Verification items for the finished model (mm, model axes). A direction names the side the tool comes from. Coordinates: 2 decimals unless noted, no trailing zeros. Order: outer loops, then holes, each group sorted by start corner. A loop starts at its lowest first (then second) coordinate and runs counter-clockwise, first axis right, second up. Notation, with made-up numbers: M 45.25,-10.5 L 84.25,-10.5 A33 ccw 84.25,20.5 Z; hole C -39,-40 d10. An arc over 180 degrees is marked long. Use one line per item in the form item = value. Start each with the question number.
```python
from build123d import *

# Parameters (mm, degrees)
F1_DEPTH = 6.35
F0_W     = 3.81
F0_H     = 76.2000009209
F0_H_2   = 76.2
F2_DEPTH = 3.175


# Not quite as in the source:
# - ends of sketch curves that miss each other by under 0.0002 mm in the source are joined


with BuildPart() as f1:
    # F0 (on Top) → F1 (new body, symmetric)
    with BuildSketch(Plane.XY):
        with BuildLine():
            Line((-49.2071506187, 28.1480993807), (-49.2071506187, 21.7980993807))
            Line((-49.2071506187, 21.7980993807), (-45.3971506187, 21.7980993807))
            Line((-45.3971506187, 21.7980993807), (-26.2557423981, 21.7980993807))
            Line((-26.2557423981, 21.7980993807), (-22.4457423981, 21.7980993807))
            Line((-22.4457423981, 21.7980993807), (-1.3203332201, 21.7980993807))
            Line((-1.3203332201, 21.7980993807), (2.4896667799, 21.7980993807))
            Line((2.4896667799, 21.7980993807), (21.6630548239, 21.7980993807))
            Line((21.6630548239, 21.7980993807), (25.4730548239, 21.7980993807))
            Line((25.4730548239, 21.7980993807), (45.6722128358, 21.7980993807))
            Line((45.6722128358, 21.7980993807), (49.4822128358, 21.7980993807))
            Line((49.4822128358, 21.7980993807), (49.8528493813, 21.7980993807))
            Line((49.8528493813, 21.7980993807), (49.8528493813, 28.1480993807))
            ThreePointArc((49.8528493813, 28.1480993807), (47.9929774418, 32.6382274413), (43.5028493813, 34.4980993807))
            Line((43.5028493813, 34.4980993807), (-42.8571506187, 34.4980993807))
            ThreePointArc((-42.8571506187, 34.4980993807), (-47.3472786793, 32.6382274413), (-49.2071506187, 28.1480993807))
        make_face()
    extrude(amount=F1_DEPTH, both=True)

    # F0 (on Top) → F2 (join, symmetric)
    with BuildSketch(Plane.XY):
        with BuildLine():
            Line((-49.2071506187, 28.1480993807), (-49.2071506187, 21.7980993807))
            Line((-49.2071506187, 21.7980993807), (-45.3971506187, 21.7980993807))
            Line((-45.3971506187, 21.7980993807), (-26.2557423981, 21.7980993807))
            Line((-26.2557423981, 21.7980993807), (-22.4457423981, 21.7980993807))
            Line((-22.4457423981, 21.7980993807), (-1.3203332201, 21.7980993807))
            Line((-1.3203332201, 21.7980993807), (2.4896667799, 21.7980993807))
            Line((2.4896667799, 21.7980993807), (21.6630548239, 21.7980993807))
            Line((21.6630548239, 21.7980993807), (25.4730548239, 21.7980993807))
            Line((25.4730548239, 21.7980993807), (45.6722128358, 21.7980993807))
            Line((45.6722128358, 21.7980993807), (49.4822128358, 21.7980993807))
            Line((49.4822128358, 21.7980993807), (49.8528493813, 21.7980993807))
            Line((49.8528493813, 21.7980993807), (49.8528493813, 28.1480993807))
            ThreePointArc((49.8528493813, 28.1480993807), (47.9929774418, 32.6382274413), (43.5028493813, 34.4980993807))
            Line((43.5028493813, 34.4980993807), (-42.8571506187, 34.4980993807))
            ThreePointArc((-42.8571506187, 34.4980993807), (-47.3472786793, 32.6382274413), (-49.2071506187, 28.1480993807))
        make_face()
        with BuildLine():
            Line((-45.3971506187, 21.7980993807), (-49.2071506187, 21.7980993807))
            Line((-49.2071506187, 21.7980993807), (-49.2071506187, -50.5919006193))
            ThreePointArc((-49.2071506187, -50.5919006193), (-48.0912274551, -53.2859774556), (-45.3971506187, -54.4019006193))
            Line((-45.3971506187, -54.4019006193), (-45.3971506187, 21.7980993807))
        make_face()
        with Locations((-24.3507423981, -16.3019010797)):
            Rectangle(F0_W, F0_H)
        with Locations((0.5846667799, -16.3019006193)):
            Rectangle(F0_W, F0_H_2)
        with Locations((23.5680548239, -16.3019006193)):
            Rectangle(F0_W, F0_H_2)
        with BuildLine():
            Line((49.4822128358, -50.5919006193), (49.4822128358, 21.7980993807))
            Line((49.4822128358, 21.7980993807), (45.6722128358, 21.7980993807))
            Line((45.6722128358, 21.7980993807), (45.6722128358, -54.4019006193))
            ThreePointArc((45.6722128358, -54.4019006193), (48.3662896722, -53.2859774556), (49.4822128358, -50.5919006193))
        make_face()
    extrude(amount=F2_DEPTH, both=True)


solid = f1.part
```
1. Tool access check on faces 1 (the flat face through (-47, -16, -3.175)), 2 (the flat face through (48, -16, 3.175)), 3 (the flat face through (49.482, -15, 0)), 4 (the flat face through (0, 28, -6.35)), 5 (the flat face through (-1.32, -17, 0)). Record the directions out of +Z, -Z, +X, -X, +Y, -Y that give a thin tool (end or side, any length) a straight path to the whole face; none if there is none.
2. Release check for a two-part mould opening along X. For faces 6 (the cylindrical face through (48.04, 32.59, 0.09)), 7 (the flat face through (1, 34.498, 0)), 8 (the flat face through (21.663, -17, 0)) record: pulls with the +X half, pulls with the -X half, needs draft (parallel to the pull), parting line crosses it, or undercut.
3. Cross-section at B-B on z = -1.25. Enter the section's corners in (x, y), and give its area (3 significant figures).
4. Cross-section at A-A on y = -26.5. Enter the section's corners in (x, z) (3 decimals), and give its area (3 significant figures).
5. Depth check by flat-ended pin: P1, Ø1.9, axis at x = 23, y = -11.5, coming from the -Z side (3 decimals); P2, Ø1.9, axis at y = -9.5, z = -0.5, coming from the +X side; P3, Ø1.1, axis at x = -48, y = -16, coming from the +Z side (3 decimals). Enter the tip coordinate at first touch or a pass-through.
6. Material ranges on line 1 along X through (y, z) = (5, 2.75); line 2 along Y through (x, z) = (-25.5, 4.5); line 3 along X through (y, z) = (29.5, -3), recorded low to high.
7. Cross-section at C-C on x = 36. Enter the section's corners in (y, z).
Final values:
q1.face_1 = -Z, +X, -X, -Y
q1.face_2 = +Z, +X, -X, -Y
q1.face_3 = +Z, -Z, +X, -Y
q1.face_4 = -Z, +X, -X, +Y, -Y
q1.face_5 = +Z, -Z, -Y
q2.face_6 = pulls with the +X half
q2.face_7 = needs draft
q2.face_8 = undercut
q3.outline = M -49.21,-50.59 A3.81 ccw -45.4,-54.4 L -45.4,21.8 L -26.26,21.8 L -26.26,-54.4 L -22.45,-54.4 L -22.45,21.8 L -1.32,21.8 L -1.32,-54.4 L 2.49,-54.4 L 2.49,21.8 L 21.66,21.8 L 21.66,-54.4 L 25.47,-54.4 L 25.47,21.8 L 45.67,21.8 L 45.67,-54.4 A3.81 ccw 49.48,-50.59 L 49.48,21.8 L 49.85,21.8 L 49.85,28.15 A6.35 ccw 43.5,34.5 L -42.86,34.5 A6.35 ccw -49.21,28.15 Z
q3.area = 2,690 mm2
q4.outline = M -49.207,-3.175 L -45.397,-3.175 L -45.397,3.175 L -49.207,3.175 Z; M -26.256,-3.175 L -22.446,-3.175 L -22.446,3.175 L -26.256,3.175 Z; M -1.32,-3.175 L 2.49,-3.175 L 2.49,3.175 L -1.32,3.175 Z; M 21.663,-3.175 L 25.473,-3.175 L 25.473,3.175 L 21.663,3.175 Z; M 45.672,-3.175 L 49.482,-3.175 L 49.482,3.175 L 45.672,3.175 Z
q4.area = 121 mm2
q5.P1 = -3.175
q5.P2 = 49.48
q5.P3 = 3.175
q6.line_1 = -49.21 to -45.4, -26.26 to -22.45, -1.32 to 2.49, 21.66 to 25.47, 45.67 to 49.48
q6.line_2 = 21.8 to 34.5
q6.line_3 = -49.06 to 49.71
q7.outline = M 21.8,-6.35 L 34.5,-6.35 L 34.5,6.35 L 21.8,6.35 Z
